Work out the finished part from the listing and answer in its coordinate system (mm). Face numbers are marked on the shaded views. A direction names the side the tool comes from. Give positions to 0.01 mm unless a question says otherwise; leave off trailing zeros. Write each loop counter-clockwise with the first axis right and the second up, starting at its lowest first coordinate (ties: lowest second). Pieces come first, ordered by that corner, then holes. Notation, with made-up numbers: (77, 80) - (103, 80) arc R21 cw to (103, 108) - close; hole circle Ø9 at (-3.5, 53). An arc over 180 degrees is marked (long way). Write item = value, one per line.
Autodesk Inventor part; units mm, degrees
ref_plane "YZ Plane" through (0, 0, 0) normal (1, 0, 0) x (0, 1, 0)
ref_plane "XZ Plane" through (0, 0, 0) normal (0, 1, 0) x (-1, 0, 0)
ref_plane "XY Plane" through (0, 0, 0) normal (0, 0, 1) x (1, 0, 0)
sketch "スケッチ1" plane through (0, 0, 0) normal (0, 1, 0) x (-1, 0, 0)
  line L0 (0, 0) -> (-20, 0)
  line L1 (-20, 0) -> (-20, 50)
  line L2 (-20, 50) -> (0, 50)
  line L3 (0, 50) -> (0, 0)
  dimension "d0" = 20
  dimension "d1" = 50
extrude "押し出し1" add sketch "スケッチ1" along normal blind 3
sketch "スケッチ2" plane through (0, 3, 0) normal (0, 1, 0) x (1, 0, 0)
  line L0 (0, -50) -> (20, -50)
  line L1 (0, 0) -> (2, 0)
  line L2 (2, 0) -> (2, -50)
  line L3 (2, -50) -> (0, -50)
  line L4 (0, -50) -> (0, 0)
  dimension "d4" = 2
extrude "押し出し2" add sketch "スケッチ2" along normal blind 30
sketch "スケッチ3" plane through (2, 3, 50) normal (1, 0, 0) x (0, 0, -1)
  line L0 (50, 0) -> (0, 0)
  line L1 (0, 0) -> (0, 30)
  line L2 (25, 0) -> (25, 17.5)
  circle A0 centre (25, 17.5) radius 3
  point P0 (50, -3)
  dimension "d7" = 17.5
  dimension "d8" = 6
hole "穴1" at (2, 20.5, 25) direction (-1, 0, 0) diameter 6 depth 8 tip angle 118
sketch "スケッチ4" plane through (0, 3, 0) normal (0, 1, 0) x (1, 0, 0)
  line L0 (20, -50) -> (20, 0)
  line L1 (20, 0) -> (2, 0)
  line L2 (20, -25) -> (6, -25)
  line L3 (6, -25) -> (6, -15)
  line L4 (6, -15) -> (6, -5)
  point P0 (0, 0)
  point P1 (6, -45)
  point P2 (6, -35)
  point P3 (6, -45)
  dimension "d16" = 14
  dimension "d17" = 10
  dimension "d18" = 10
hole "穴2" at (6, 3, 5) at (6, 3, 15) at (6, 3, 25) at (6, 3, 35) at (6, 3, 45) direction (0, -1, 0) diameter 3 depth 8 tip angle 118
properties part number "知能ロボコンＬ字"
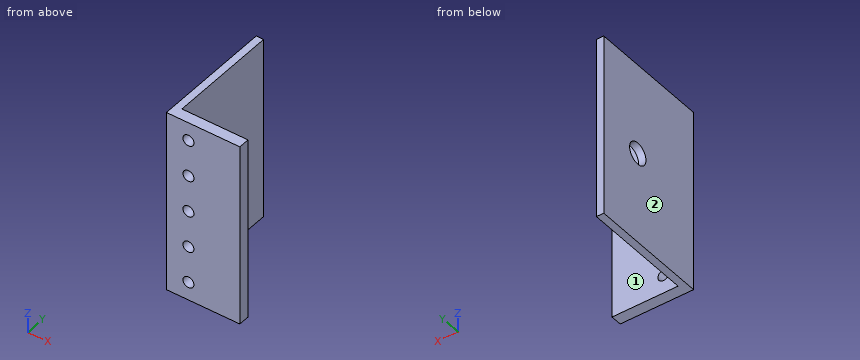
1. Straight lines are drawn through the part: line 1 (Z direction, x = 6, y = 0.85); line 2 (X direction, y = 2, z = 25); line 3 (Y direction, x = 1.55, z = 25). For each, find the intervals that lie inside material, in ascending order.
Solution:
line_1 = 0 to 3.5, 6.5 to 13.5, 16.5 to 23.5, 26.5 to 33.5, 36.5 to 43.5, 46.5 to 50
line_2 = 0 to 4.5, 7.5 to 20
line_3 = 0 to 17.5, 23.5 to 33
2. A tool of negligible diameter and unlimited length cuts with its end or side. For the marked faces 1 and 2, from which of +Z, -Z, +X, -X, +Y, -Y can it reach the whole face along a straight path? Write none if from no direction.
Solution:
face_1 = +Z, -Z, +X, +Y
face_2 = +Z, -Z, -X, +Y, -Y
3. Find section A-A, the plane z = 5. Give the vertices of the cut face in (x, y).
Solution:
outline = (0, 0) - (4.5, 0) - (4.5, 3) - (2, 3) - (2, 33) - (0, 33) - close; (7.5, 0) - (20, 0) - (20, 3) - (7.5, 3) - close
4. Find section C-C, the plane x = 6. Give the vertices of the cut face in (y, z), then the cut area to 3 significant figures.
Solution:
outline = (0, 0) - (3, 0) - (3, 3.5) - (0, 3.5) - close; (0, 6.5) - (3, 6.5) - (3, 13.5) - (0, 13.5) - close; (0, 16.5) - (3, 16.5) - (3, 23.5) - (0, 23.5) - close; (0, 26.5) - (3, 26.5) - (3, 33.5) - (0, 33.5) - close; (0, 36.5) - (3, 36.5) - (3, 43.5) - (0, 43.5) - close; (0, 46.5) - (3, 46.5) - (3, 50) - (0, 50) - close
area = 105 mm^2
5. Find section D-D, the plane z = 25. Give the vertices of the cut face in (x, y), then the cut area to 3 significant figures.
Solution:
outline = (0, 0) - (4.5, 0) - (4.5, 3) - (2, 3) - (2, 17.5) - (0, 17.5) - close; (0, 23.5) - (2, 23.5) - (2, 33) - (0, 33) - close; (7.5, 0) - (20, 0) - (20, 3) - (7.5, 3) - close
area = 99.0 mm^2
6. Given pin 1 (1.5 mm diameter, centred on x = 6.5, z = 18, fed in from -Y); pin 2 (5 mm diameter, centred on y = 20.5, z = 25, fed in from -X); pin 3 (4 mm diameter, centred on y = 9.5, z = 30, fed in from +X); pin 4 (5.5 mm diameter, centred on x = 13, z = 33.5, fed in from +Y), each flat-ended and moving along its own axis, determine where each tip first touches the part or whether it passes through.
Solution:
pin_1 = 0
pin_2 = through
pin_3 = 2
pin_4 = 3
7. Find section B-B, the plane y = 20.5. Give the vertices of the cut face in (x, z).
Solution:
outline = (0, 0) - (2, 0) - (2, 22) - (0, 22) - close; (0, 28) - (2, 28) - (2, 50) - (0, 50) - close
